```python
from build123d import *

# Parameters (mm, degrees)
EXTRUDE_1_DEPTH     = 3
FILLET_1_R          = 1.27
SKETCH_2_W          = 2.88
SKETCH_2_H          = 29.994
CUT_EXTRUDE_1_DEPTH = 3


with BuildPart() as part:
    # 스케치1 → 보스-돌출1 (new body)
    with BuildSketch(Plane.XY):
        Polygon((-3, 33.044), (3, 33.044), (3, -23.944), (6, -23.944), (6, -33.044), (3, -33.044), (3, -26.944), (-3, -26.944), (-3, -33.044), (-6, -33.044), (-6, -23.944), (-3, -23.944), align=None)
    extrude(amount=EXTRUDE_1_DEPTH)

    # 필렛1
    fillet_1_edges = [part.edges().sort_by_distance(p)[0] for p in [
        (6, -23.944, 1.5),
        (-6, -23.944, 1.5),
    ]]
    fillet(fillet_1_edges, radius=FILLET_1_R)

    # 스케치2 → 컷-돌출1 (cut)
    with BuildSketch(Plane(origin=(0, 0, 0), x_dir=(-1, 0, 0), z_dir=(0, 0, -1))):
        with Locations((0, -11.947)):
            Rectangle(SKETCH_2_W, SKETCH_2_H)
    extrude(amount=-CUT_EXTRUDE_1_DEPTH, mode=Mode.SUBTRACT)


solid = part.part
```
For this review, take the finished solid that the model builds, in its own axes (mm). A direction names the side the tool comes from. Round coordinates to 2 decimals unless told otherwise and drop trailing zeros. Write each loop counter-clockwise with the first axis right and the second up, starting at its lowest first coordinate (ties: lowest second). Pieces come first, ordered by that corner, then holes. Notation, with made-up numbers: (26, 12) - (56, 12) arc R17 cw to (56, 28) - close; hole circle Ø5 at (-26, 73.25). An arc over 180 degrees is marked (long way). Answer as a JSON object with one key per item and string values.
1. We need section D-D on y = 8. Give the boundary of the cut face in (x, z).
Response values:
{"outline": "(-3, 0) - (3, 0) - (3, 3) - (-3, 3) - close"}
2. We need section C-C on x = -3.75. Give the boundary of the cut face in (y, z), then the cut area to 3 significant figures.
Response values:
{"outline": "(-33.04, 0) - (-23.94, 0) - (-23.94, 3) - (-33.04, 3) - close", "area": "27.3 mm2"}
3. To check wall thickness, follow line 1 along X through (y, z) = (-8.5, 2.7); line 2 along X through (y, z) = (-26, 1.35); line 3 along Y through (x, z) = (1.75, 2.8). State the ranges of each line that lie inside material, in increasing order.
Response values:
{"line 1": "x = -3 to -1.44, 1.44 to 3", "line 2": "x = -6 to -1.44, 1.44 to 6", "line 3": "y = -26.94 to 33.04"}
4. For pin 1 Ø1.5 at (x, y) = (0.5, -2.5) entering from +Z; pin 2 Ø0.5 at (x, z) = (-4, 1.5) entering from +Y; pin 3 Ø0.9 at (y, z) = (-9, 2) entering from -X; pin 4 Ø0.5 at (x, z) = (-2.5, 1.5) entering from -Y, all flat-tipped, find the tip position at first contact; note any pin that passes through.
Response values:
{"pin 1": "passes through", "pin 2": "stops at y = -23.94", "pin 3": "stops at x = -3", "pin 4": "stops at y = -26.94"}
5. We need section A-A on y = -28. Give the boundary of the cut face in (x, z), then the cut area to 3 significant figures.
Response values:
{"outline": "(-6, 0) - (-3, 0) - (-3, 3) - (-6, 3) - close; (3, 0) - (6, 0) - (6, 3) - (3, 3) - close", "area": "18.0 mm2"}
6. Tool access review of faces 1 (the face through (2, -26.944, 1)), 2 (the face through (4, -23.944, 1)), 3 (the face through (5, -33.044, 1)), 4 (the face through (0, 33.044, 1)), 5 (the face through (-4, -23.944, 1)): name each direction out of +Z, -Z, +X, -X, +Y, -Y from which nothing blocks a thin tool from reaching the whole face with its end or side.
Response values:
{"face 1": "+Z, -Z, -Y", "face 2": "+Z, -Z, +X, +Y", "face 3": "+Z, -Z, +X, -X, -Y", "face 4": "+Z, -Z, +X, -X, +Y", "face 5": "+Z, -Z, -X, +Y"}
7. Draft analysis for pull direction X (two halves, no side actions). For faces 6 (the face through (3, -30, 1)), 7 (the face through (-3, 4, 1)), 8 (the face through (0, 8, 0)), 9 (the face through (5.62, -24.31, 1.52)), state which applies: +X half, -X half, draft (parallel to the pull), parting line (faces both ways), or undercut.
Response values:
{"face 6": "undercut", "face 7": "-X half", "face 8": "draft", "face 9": "+X half"}
8. We need section B-B on z = 0.7. Give the boundary of the cut face in (x, y), then the cut area to 3 significant figures.
Response values:
{"outline": "(-6, -33.04) - (-3, -33.04) - (-3, -26.94) - (-1.44, -26.94) - (-1.44, 3.05) - (1.44, 3.05) - (1.44, -26.94) - (3, -26.94) - (3, -33.04) - (6, -33.04) - (6, -25.21) arc R1.27 ccw to (4.73, -23.94) - (3, -23.94) - (3, 33.04) - (-3, 33.04) - (-3, -23.94) - (-4.73, -23.94) arc R1.27 ccw to (-6, -25.21) - close", "area": "327 mm2"}
